The figure shows three views and two pictorial views of one solid part (mm, origin at its lowest corner). Answer the questions. Coordinates: 2 decimals unless noted, no trailing zeros. Write each loop counter-clockwise with the first axis right and the second up, starting at its lowest first coordinate (ties: lowest second). Pieces come first, ordered by that corner, then holes. Notation, with made-up numbers: M 64.5,-0.5 L 96.5,-0.5 A22 ccw 96.5,11.5 Z; hole C -4.5,4.5 d2. An arc over 180 degrees is marked long. Answer as CSV lines item,"result".
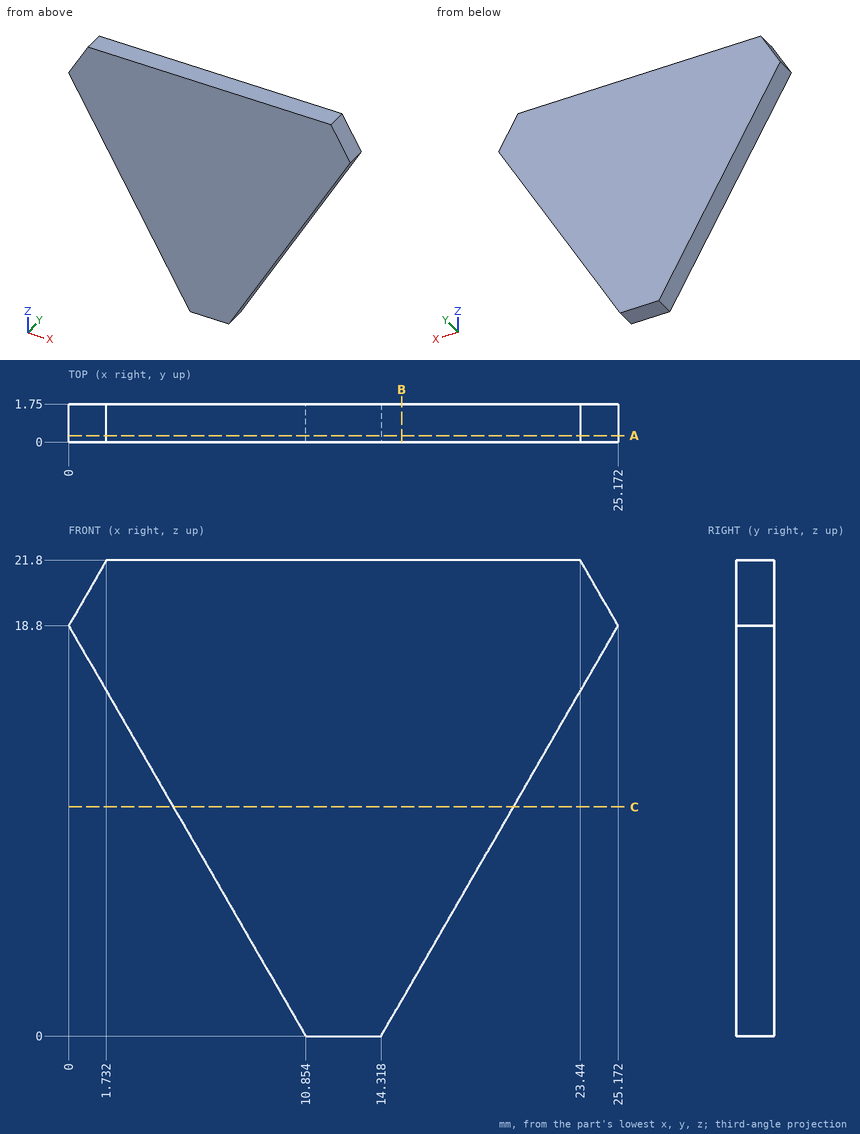
Q1. Find section B-B (x = 15.25). Give the vertices of the cut face in (y, z).
Output:
outline,"M 0,1.61 L 1.75,1.61 L 1.75,21.8 L 0,21.8 Z"
Q2. Find section A-A (y = 0.3). Give the vertices of the cut face in (x, z).
Output:
outline,"M 0,18.8 L 10.85,0 L 14.32,0 L 25.17,18.8 L 23.44,21.8 L 1.73,21.8 Z"
Q3. Straight lines are drawn through the part: line 1 (Z direction, x = 2.25, y = 1.35) (1 decimal); line 2 (Z direction, x = 4.75, y = 0.5) (1 decimal); line 3 (X direction, y = 0.3, z = 7.25) (1 decimal). For each, find the intervals that lie inside material, in ascending order.
Output:
line 1,"14.9 to 21.8"
line 2,"10.6 to 21.8"
line 3,"6.7 to 18.5"
Q4. Find section C-C (z = 10.5). Give the vertices of the cut face in (x, y).
Output:
outline,"M 4.79,0 L 20.38,0 L 20.38,1.75 L 4.79,1.75 Z"
